The model under review builds one solid part; all positions refer to its coordinate system, in mm. Face numbers are marked on the shaded views. A direction names the side the tool comes from. Coordinates: 2 decimals unless noted, no trailing zeros. Write each loop counter-clockwise with the first axis right and the second up, starting at its lowest first coordinate (ties: lowest second). Pieces come first, ordered by that corner, then holes. Notation, with made-up numbers: (27.25, 0.5) -> (86.25, 0.5) arc R5 ccw to (86.25, 7.5) -> close; hole circle Ø8 at (-36.5, 1). An arc over 180 degrees is marked (long way). Write each question's results on one line, items separated by ' | '.
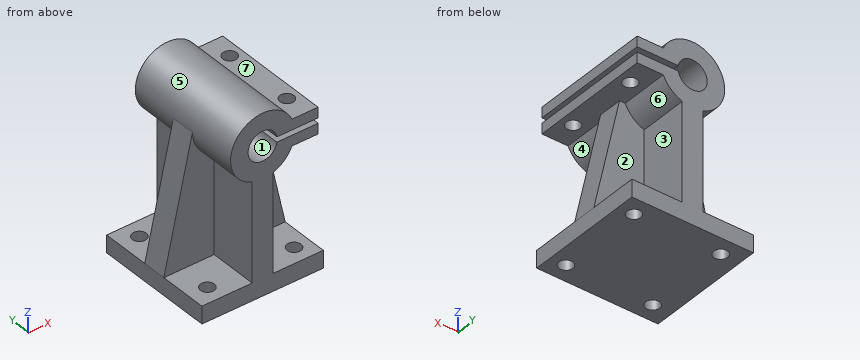
```python
from build123d import *

# Parameters (mm, degrees)
SZKIC2_W                    = 35
SZKIC2_H                    = 5
DODANIE_WYCI_GNI_CIE1_DEPTH = 35
SZKIC3_R                    = 9.25
SZKIC3_R_2                  = 4.2
DODANIE_WYCI_GNI_CIE2_DEPTH = 35
SZKIC4_W                    = 6
SZKIC4_H                    = 30.71029356
DODANIE_WYCI_GNI_CIE3_DEPTH = 35
DODANIE_WYCI_GNI_CIE4_START = -14
DODANIE_WYCI_GNI_CIE4_DEPTH = 7
WYTNIJ_WYCI_GNI_CIE1_REACH  = 66.481
SZKIC7_R                    = 2
WYTNIJ_WYCI_GNI_CIE2_REACH  = 62.583
SZKIC8_W                    = 10.637888195
SZKIC8_H                    = 1.500000817
SZKIC11_W                   = 9.672485651
SZKIC11_H                   = 3
SZKIC11_H_2                 = 2.999999183
DODANIE_WYCI_GNI_CIE6_DEPTH = 35
SZKIC12_R                   = 2
WYTNIJ_WYCI_GNI_CIE4_DEPTH  = 12


with BuildPart() as part:
    # Szkic2 → Dodanie-wyci_gni_cie1 (new body)
    with BuildSketch(Plane(origin=(0, 0, 0), x_dir=(1, 0, 0), z_dir=(0, 1, 0))):
        with Locations((0, 2.5)):
            Rectangle(SZKIC2_W, SZKIC2_H)
    extrude(amount=DODANIE_WYCI_GNI_CIE1_DEPTH)



with BuildPart() as body_2:
    # Szkic3 → Dodanie-wyci_gni_cie2 (new body)
    with BuildSketch(Plane.XZ):
        with Locations(Location((0, 37, 0), (0, 0, 270))):
            Circle(SZKIC3_R)
        with Locations(Location((0, 37, 0), (0, 0, 270))):
            Circle(SZKIC3_R_2, mode=Mode.SUBTRACT)
    extrude(amount=-DODANIE_WYCI_GNI_CIE2_DEPTH)


with BuildPart() as part_1:
    add(part.part)

    add(body_2.part)  # Dodanie-wyci_gni_cie3 merges body 2
    # Szkic4 → Dodanie-wyci_gni_cie3 (add)
    with BuildSketch(Plane.XZ):
        with Locations((0, 15.35514678)):
            Rectangle(SZKIC4_W, SZKIC4_H)
    extrude(amount=-DODANIE_WYCI_GNI_CIE3_DEPTH)

    # Szkic5 → Dodanie-wyci_gni_cie4 (add)
    with BuildSketch(Plane.XZ.offset(DODANIE_WYCI_GNI_CIE4_START)):
        Polygon((0, 0), (-17.5, 0), (-9.25, 37), (-3, 28.25), align=None)
        Polygon((3, 0), (3, 28.25), (9.25, 37), (17.5, 0), align=None)
    extrude(amount=-DODANIE_WYCI_GNI_CIE4_DEPTH)

    # Szkic7 → Wytnij-wyci_gni_cie1 (cut, up to next)
    with BuildSketch(Plane(origin=(0, 0, -5), x_dir=(-1, 0, 0), z_dir=(0, 0, -1)), mode=Mode.PRIVATE) as wytnij_wyci_gni_cie1_sk1:
        with Locations((-13, 30)):
            Circle(SZKIC7_R)
    wytnij_wyci_gni_cie1_tool1 = extrude(wytnij_wyci_gni_cie1_sk1.sketch, amount=-WYTNIJ_WYCI_GNI_CIE1_REACH, mode=Mode.PRIVATE) & part_1.part
    # Szkic7 → Wytnij-wyci_gni_cie1 (cut, up to next)
    with BuildSketch(Plane(origin=(0, 0, -5), x_dir=(-1, 0, 0), z_dir=(0, 0, -1)), mode=Mode.PRIVATE) as wytnij_wyci_gni_cie1_sk2:
        with Locations((12, 30)):
            Circle(SZKIC7_R)
    wytnij_wyci_gni_cie1_tool2 = extrude(wytnij_wyci_gni_cie1_sk2.sketch, amount=-WYTNIJ_WYCI_GNI_CIE1_REACH, mode=Mode.PRIVATE) & part_1.part
    # Szkic7 → Wytnij-wyci_gni_cie1 (cut, up to next)
    with BuildSketch(Plane(origin=(0, 0, -5), x_dir=(-1, 0, 0), z_dir=(0, 0, -1)), mode=Mode.PRIVATE) as wytnij_wyci_gni_cie1_sk3:
        with Locations((12, 5)):
            Circle(SZKIC7_R)
    wytnij_wyci_gni_cie1_tool3 = extrude(wytnij_wyci_gni_cie1_sk3.sketch, amount=-WYTNIJ_WYCI_GNI_CIE1_REACH, mode=Mode.PRIVATE) & part_1.part
    # Szkic7 → Wytnij-wyci_gni_cie1 (cut, up to next)
    with BuildSketch(Plane(origin=(0, 0, -5), x_dir=(-1, 0, 0), z_dir=(0, 0, -1)), mode=Mode.PRIVATE) as wytnij_wyci_gni_cie1_sk4:
        with Locations((-13, 5)):
            Circle(SZKIC7_R)
    wytnij_wyci_gni_cie1_tool4 = extrude(wytnij_wyci_gni_cie1_sk4.sketch, amount=-WYTNIJ_WYCI_GNI_CIE1_REACH, mode=Mode.PRIVATE) & part_1.part
    add(wytnij_wyci_gni_cie1_tool1.solids().sort_by_distance((13, 30, -5))[0], mode=Mode.SUBTRACT)
    add(wytnij_wyci_gni_cie1_tool2.solids().sort_by_distance((-12, 30, -5))[0], mode=Mode.SUBTRACT)
    add(wytnij_wyci_gni_cie1_tool3.solids().sort_by_distance((-12, 5, -5))[0], mode=Mode.SUBTRACT)
    add(wytnij_wyci_gni_cie1_tool4.solids().sort_by_distance((13, 5, -5))[0], mode=Mode.SUBTRACT)

    # Szkic8 → Wytnij-wyci_gni_cie2 (cut, up to next)
    with BuildSketch(Plane.XZ, mode=Mode.PRIVATE) as wytnij_wyci_gni_cie2_sk1:
        with Locations((9.451437144, 37.000000409)):
            Rectangle(SZKIC8_W, SZKIC8_H)
    wytnij_wyci_gni_cie2_tool1 = extrude(wytnij_wyci_gni_cie2_sk1.sketch, amount=-WYTNIJ_WYCI_GNI_CIE2_REACH, mode=Mode.PRIVATE) & part_1.part
    add(wytnij_wyci_gni_cie2_tool1.solids().sort_by_distance((9.451437, 0, 37))[0], mode=Mode.SUBTRACT)

    # Szkic11 → Dodanie-wyci_gni_cie6 (add)
    with BuildSketch(Plane(origin=(0, 0, 0), x_dir=(-1, 0, 0), z_dir=(0, -1, 0))):
        with Locations((-11.163757175, -34.75)):
            Rectangle(SZKIC11_W, SZKIC11_H)
        with Locations((-11.163757175, -39.250000409)):
            Rectangle(SZKIC11_W, SZKIC11_H_2)
    extrude(amount=-DODANIE_WYCI_GNI_CIE6_DEPTH)

    # Szkic12 → Wytnij-wyci_gni_cie4 (cut)
    with BuildSketch(Plane.XY.offset(40.75)):
        with Locations((12.5, 28)):
            Circle(SZKIC12_R)
        with Locations((12.5, 7)):
            Circle(SZKIC12_R)
    extrude(amount=-WYTNIJ_WYCI_GNI_CIE4_DEPTH, mode=Mode.SUBTRACT)


solid = part_1.part
```
Q1. Add section C-C (z = 31). Write out the cut boundary in (x, y), plus the area to 3 significant figures.
Solution:
outline: (-10.59, 14) -> (-7.04, 14) -> (-7.04, 0) -> (7.04, 0) -> (7.04, 14) -> (10.59, 14) -> (10.59, 21) -> (7.04, 21) -> (7.04, 35) -> (-7.04, 35) -> (-7.04, 21) -> (-10.59, 21) -> close | area: 542 mm²
Q2. Add section A-A (x = 0). Write out the cut boundary in (y, z).
Solution:
outline: (0, -5) -> (35, -5) -> (35, 32.8) -> (0, 32.8) -> close; (0, 41.2) -> (35, 41.2) -> (35, 46.25) -> (0, 46.25) -> close
Q3. Draft analysis for pull direction X (two halves, no side actions). For the marked faces 1, 2 and 3, state which applies: pulls with the +X half, pulls with the -X half, needs draft (parallel to the pull), parting line crosses it, or undercut.
Solution:
face 1: undercut | face 2: needs draft | face 3: pulls with the +X half
Q4. Clearance check with flat-ended pins moving along their axes: P1, Ø6, axis at x = -10.5, y = 24.5, coming from the +Z side; P2, Ø0.9, axis at y = 23, z = 35.5, coming from the +X side; P3, Ø11, axis at y = 29, z = 9, coming from the -X side. State where each tip first meets the part, or that it passes through.
Solution:
P1: z = 42.41 | P2: x = 16 | P3: x = -3
Q5. Add section B-B (y = 27). Write out the cut boundary in (x, z).
Solution:
outline: (-17.5, -5) -> (17.5, -5) -> (17.5, 0) -> (3, 0) -> (3, 28.25) arc R9.25 ccw to (8.46, 33.25) -> (10.77, 33.25) -> (10.77, 36.25) -> (4.13, 36.25) arc R4.2 cw (long way) to (4.13, 37.75) -> (10.77, 37.75) -> (10.77, 40.75) -> (8.46, 40.75) arc R9.25 ccw (long way) to (-3, 28.25) -> (-3, 0) -> (-17.5, 0) -> close; (14.23, 33.25) -> (16, 33.25) -> (16, 36.25) -> (14.23, 36.25) -> close; (14.23, 37.75) -> (16, 37.75) -> (16, 40.75) -> (14.23, 40.75) -> close
Q6. For line 1 (Y direction, x = -12, z = -1); line 2 (X direction, y = 25, z = 6); line 3 (Y direction, x = -9, z = 18), list the stretches that pass through material, from the lowest coordinate up. Write a range as from..to.
Solution:
line 1: 0..3, 7..28, 32..35 | line 2: -3..3 | line 3: 14..21
Q7. Add section D-D (y = 16). Write out the cut boundary in (x, z), plus the area to 3 significant figures.
Solution:
outline: (-17.5, -5) -> (17.5, -5) -> (17.5, 0) -> (10.09, 33.25) -> (16, 33.25) -> (16, 36.25) -> (4.13, 36.25) arc R4.2 cw (long way) to (4.13, 37.75) -> (16, 37.75) -> (16, 40.75) -> (8.46, 40.75) arc R9.25 ccw to (-9.25, 37) -> (-17.5, 0) -> close | area: 1,280 mm²
Q8. Machinability: for the marked faces 4, 5, 6 and 7, which of the approach directions +Z, -Z, +X, -X, +Y, -Y give a long, thin tool a straight path to every point of the face, cutting with its end or side? Answer none if there is none.
Solution:
face 4: +X, -Y | face 5: none | face 6: +X, +Y | face 7: +Z, +X, +Y, -Y
